```python
from build123d import *

# Parameters (mm, degrees)
F0_W     = 76.2
F0_H     = 107.95
F0_R     = 11.1125
F1_DEPTH = 12.7
F2_W     = 69.85
F2_H     = 50.8
F3_DEPTH = 6.35
F4_START = -69.85
F4_DEPTH = 6.35


with BuildPart() as f1:
    # F0 (on Front) → F1 (new body)
    with BuildSketch(Plane.XZ):
        Rectangle(F0_W, F0_H)
        with Locations((0, -15.875)):
            Circle(F0_R, mode=Mode.SUBTRACT)
    extrude(amount=F1_DEPTH)

    # F2 (on face) → F3 (join)
    with BuildSketch(Plane.YZ.offset(38.1)):
        with Locations((34.925, -28.575)):
            Rectangle(F2_W, F2_H)
    extrude(amount=-F3_DEPTH)

    # F2 (on face) → F4 (join)
    with BuildSketch(Plane.YZ.offset(38.1).offset(F4_START)):
        with Locations((34.925, -28.575)):
            Rectangle(F2_W, F2_H)
    extrude(amount=-F4_DEPTH)


solid = f1.part
```
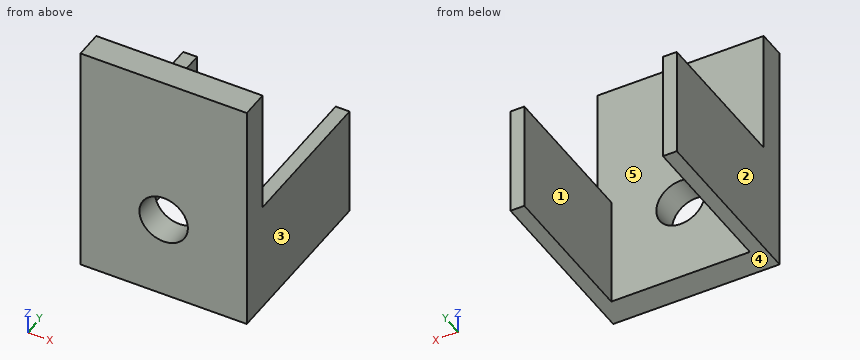
Part model, mm, in its own coordinate system. Face numbers are marked on the shaded views. A direction names the side the tool comes from. Coordinates: 2 decimals unless noted, no trailing zeros. Order: outer loops, then holes, each group sorted by start corner. A loop starts at its lowest first (then second) coordinate and runs counter-clockwise, first axis right, second up. Notation, with made-up numbers: (62.5, 40.5) - (109.5, 40.5) arc R10 cw to (109.5, 55.5) - close; hole circle Ø7 at (2.5, -27). An arc over 180 degrees is marked (long way). Return JSON: item names as keys, results as strings. Group by question number.
Item 1: Pull direction X, two halves, no side cores. Call the marked faces 3, 4 and 5: pulls with the +X half, pulls with the -X half, needs draft (parallel to the pull), parting line crosses it, or undercut.
Item 2: Cut at B-B (x = 0). List the corners of the cut face in (y, z) (1 decimal).
Item 3: Cut at C-C (z = -34.5). List the corners of the cut face in (x, y), plus the area to 3 significant figures.
Item 4: Cut at A-A (y = 62). List the corners of the cut face in (x, z) (3 decimals).
Item 5: Which spindle directions (+Z, -Z, +X, -X, +Y, -Y) get a long thin tool onto all of the face, cutting with end or side? Do the marked faces 1 and 2. Say none if no direction does.
Item 6: Pin check, flat tips, straight feed: pin 1 (3 mm diameter, centred on x = 35, y = 24.5, fed in from +Z) (3 decimals); pin 2 (23 mm diameter, centred on x = 5, z = 4, fed in from +Y); pin 3 (5 mm diameter, centred on y = 52.5, z = 0, fed in from +X). Stop position of each tip, or through.
Item 7: Cut at D-D (y = -3). List the corners of the cut face in (x, z) (1 decimal).
Item 8: Drill centre lines: probe 1 along Z at (x, y) = (0, -7) (1 decimal); probe 2 along X at (y, z) = (55, -36); probe 3 along Y at (x, z) = (-26, -28). Where is each one in solid material? Low to high. Write a range as from..to.
Check values:
{
 "1": {"face 3": "pulls with the +X half", "face 4": "needs draft", "face 5": "undercut"},
 "2": {"outline": "(-12.7, -54) - (0, -54) - (0, -27) - (-12.7, -27) - close; (-12.7, -4.8) - (0, -4.8) - (0, 54) - (-12.7, 54) - close"},
 "3": {"outline": "(-38.1, -12.7) - (38.1, -12.7) - (38.1, 69.85) - (31.75, 69.85) - (31.75, 0) - (-31.75, 0) - (-31.75, 69.85) - (-38.1, 69.85) - close", "area": "1,850 mm2"},
 "4": {"outline": "(-38.1, -53.975) - (-31.75, -53.975) - (-31.75, -3.175) - (-38.1, -3.175) - close; (31.75, -53.975) - (38.1, -53.975) - (38.1, -3.175) - (31.75, -3.175) - close"},
 "5": {"face 1": "+Z, -Z, +Y", "face 2": "+Z, -Z, -X, +Y, -Y"},
 "6": {"pin 1": "stops at z = -3.175", "pin 2": "stops at y = 0", "pin 3": "passes through"},
 "7": {"outline": "(-38.1, -54) - (38.1, -54) - (38.1, 54) - (-38.1, 54) - close; hole circle Ø22.2 at (0, -15.9)"},
 "8": {"probe 1": "z = -54..-27, -4.8..54", "probe 2": "x = -38.1..-31.75, 31.75..38.1", "probe 3": "y = -12.7..0"}
}
